from build123d import *

# Parameters (mm, degrees)
F1_DEPTH = 25.4
F3_D     = 12.7
F4_W     = 94.8301074147
F4_H     = 68.1190363509
F5_DEPTH = 3.81
F6_W     = 94.6228546143
F6_H     = 76.2625485659
F7_DEPTH = 3.81


with BuildPart() as f1:
    # F0 (on Top) → F1 (new body)
    with BuildSketch(Plane.XY):
        Polygon((69.3474411964, -42.1580038965), (92.0092580879, -31.9088696007), (92.0092580879, -16.3924994838), (41.2310734391, -16.3924994838), (41.2310734391, -12.5824994838), (41.2310734391, -8.7724994838), (92.0092580879, -8.7724994838), (92.0092580879, 7.7151303993), (69.3474411964, 17.9642646951), (6.6018956661, 17.9642646951), (6.6018956661, 7.7151303993), (-31.4981043339, 7.7151303993), (-31.4981043339, -2.4448696007), (-12.4481043339, -2.4448696007), (6.6018956661, -2.4448696007), (6.6018956661, -21.7488696007), (-31.4981043339, -21.7488696007), (-31.4981043339, -31.9088696007), (6.6018956661, -31.9088696007), (6.6018956661, -42.1580038965), align=None)
    extrude(amount=F1_DEPTH)

    # F3 (through all)
    with Locations(Plane(origin=(0, 7.7151303993, 0), x_dir=(-1, 0, 0), z_dir=(0, 1, 0))):
        with Locations((12.0056932792, 11.6236191243)):
            Hole(F3_D / 2)

    # F4 (on face) → F5 (cut)
    with BuildSketch(Plane.XY.offset(25.4)):
        with Locations((54.0169493735, -16.0952534803)):
            Rectangle(F4_W, F4_H)
    extrude(amount=-F5_DEPTH, mode=Mode.SUBTRACT)

    # F6 (on face) → F7 (cut)
    with BuildSketch(Plane(origin=(0, 0, 0), x_dir=(1, 0, 0), z_dir=(0, 0, -1))):
        with Locations((53.9133229733, 4.0267296135)):
            Rectangle(F6_W, F6_H)
    extrude(amount=-F7_DEPTH, mode=Mode.SUBTRACT)


solid = f1.part
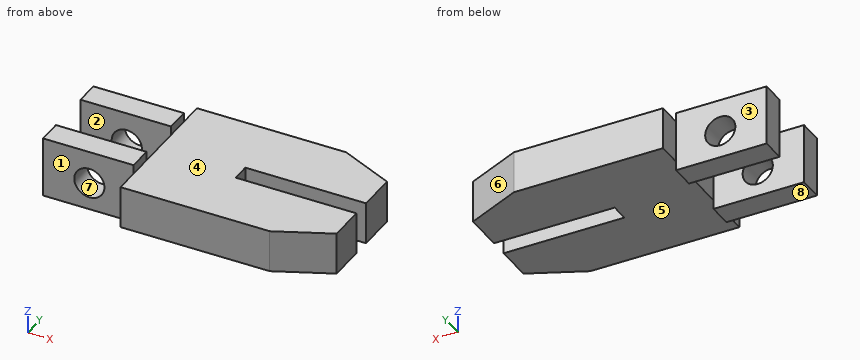
Part model, mm, in its own coordinate system. Face numbers are marked on the shaded views. A direction names the side the tool comes from. Coordinates: 2 decimals unless noted, no trailing zeros. Write each loop counter-clockwise with the first axis right and the second up, starting at its lowest first coordinate (ties: lowest second). Pieces come first, ordered by that corner, then holes. Notation, with made-up numbers: M 48,33 L 74,33 A18 ccw 74,54 Z; hole C 10.25,75 d9. An arc over 180 degrees is marked long. Return JSON: item names as keys, results as strings.
1. Saw through at C-C, the plane z = 15.25. Write the cut outline in (x, y), then the cut area to 3 significant figures.
Determined:
{"outline": "M -31.5,-31.91 L -17.22,-31.91 L -17.22,-21.75 L -31.5,-21.75 Z; M -31.5,-2.44 L -17.22,-2.44 L -17.22,7.72 L -31.5,7.72 Z; M -6.79,-31.91 L 6.6,-31.91 L 6.6,-42.16 L 69.35,-42.16 L 92.01,-31.91 L 92.01,-16.39 L 41.23,-16.39 L 41.23,-8.77 L 92.01,-8.77 L 92.01,7.72 L 69.35,17.96 L 6.6,17.96 L 6.6,7.72 L -6.79,7.72 L -6.79,-2.44 L 6.6,-2.44 L 6.6,-21.75 L -6.79,-21.75 Z", "area": "5,080 mm²"}
2. 3-axis set-ups, long thin cutter, end or side, ignore diameter. For the marked faces 1, 2, 3, 4 and 5: which of +Z, -Z, +X, -X, +Y, -Y reach the whole face in a straight line?
Determined:
{"face 1": "+Z, -Z, -X, -Y", "face 2": "+Z, -Z, -X", "face 3": "+Z, -Z, -X, +Y", "face 4": "+Z, +X, +Y, -Y", "face 5": "-Z, +X, +Y, -Y"}
3. Saw through at D-D, the plane y = -19.5. Write the cut outline in (x, z).
Determined:
{"outline": "M 6.6,3.81 L 92.01,3.81 L 92.01,21.59 L 6.6,21.59 Z"}
4. Saw through at A-A, the plane x = 5. Write the cut outline in (y, z).
Determined:
{"outline": "M -31.91,0 L -21.75,0 L -21.75,25.4 L -31.91,25.4 Z; M -2.44,0 L 7.72,0 L 7.72,25.4 L -2.44,25.4 Z"}
5. Saw through at B-B, the plane z = 2.5. Write the cut outline in (x, y).
Determined:
{"outline": "M -31.5,-31.91 L 6.6,-31.91 L 6.6,-21.75 L -31.5,-21.75 Z; M -31.5,-2.44 L 6.6,-2.44 L 6.6,7.72 L -31.5,7.72 Z"}
6. Flat gauge pins, fed straight in: pin 1 Ø10 at (x, y) = (45, 9.5) entering from +Z; pin 2 Ø1.1 at (y, z) = (1, 23.5) entering from +X; pin 3 Ø4 at (y, z) = (-14, 16.5) entering from +X; pin 4 Ø7.5 at (x, z) = (-12.01, 11.62) entering from +Y (3 decimals). Where does each tip first touch, or does it go through?
Determined:
{"pin 1": "z = 21.59", "pin 2": "x = 6.6", "pin 3": "x = 41.23", "pin 4": "through"}
7. Pull direction X, two halves, no side cores. Call the marked faces 6, 7 and 8: pulls with the +X half, pulls with the -X half, needs draft (parallel to the pull), parting line crosses it, or undercut.
Determined:
{"face 6": "pulls with the +X half", "face 7": "undercut", "face 8": "needs draft"}
8. Probe L1, parallel to Y at x = 1, z = 14.25; L2, parallel to Y at x = 68, z = 16.75; L3, parallel to Z at x = 17, y = -18. List the from-to ranges inside material, lowest first.
Determined:
{"L1": "-31.91 to -21.75, -2.44 to 7.72", "L2": "-42.16 to -16.39, -8.77 to 17.96", "L3": "3.81 to 21.59"}
